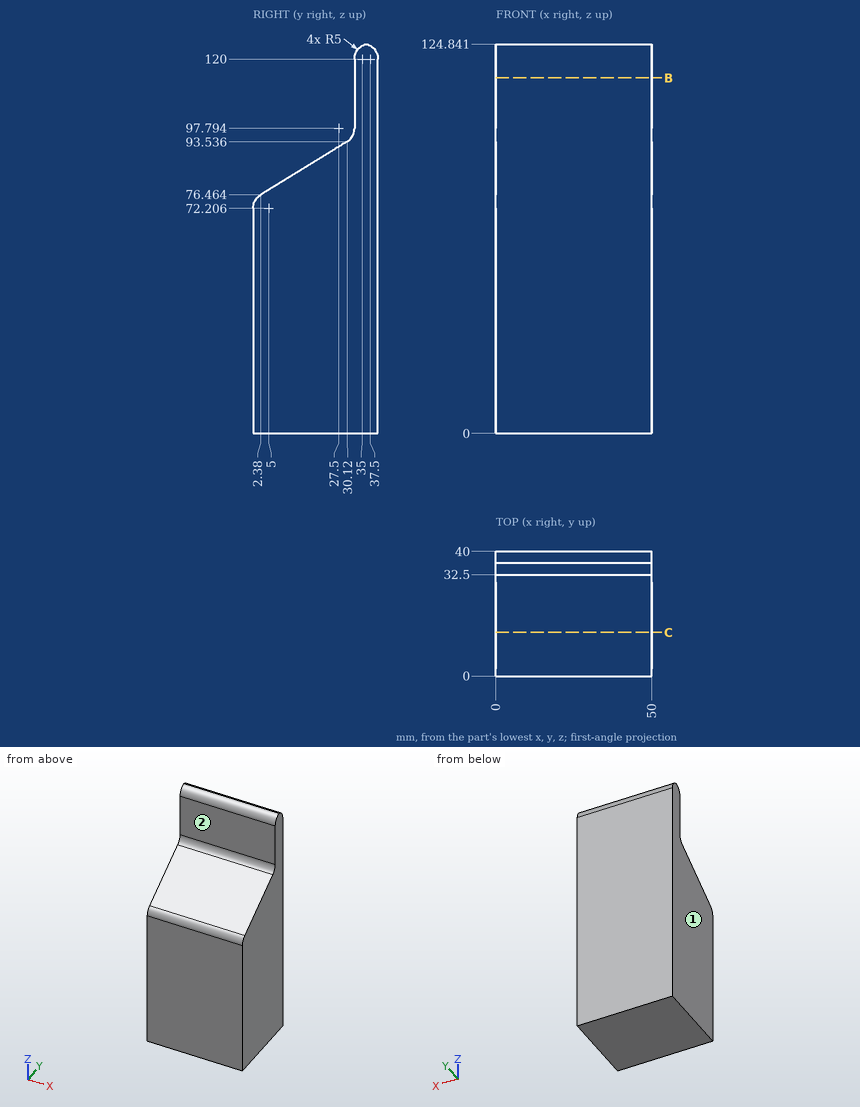
Job drawing, mm, ordinate dimensions from the low corner. One solid piece. A direction names the side the tool comes from. Round coordinates to 2 decimals unless told otherwise and drop trailing zeros. Loops run counter-clockwise (first coordinate to the right, second up) from the corner with the lowest first, then second, coordinate; pieces in that order, holes last. Notation, with made-up numbers: M -36,36.5 L -19,36.5 A13 cw -19,58.5 Z; hole C -22,73.5 d11. An arc over 180 degrees is marked long. Answer as CSV lines item,"result".
1. Cut at B-B on z = 114. Write the cut outline in (x, y).
Resolved:
outline,"M 0,32.5 L 50,32.5 L 50,40 L 0,40 Z"
2. Flat gauge pins, fed straight in: P1, Ø10, axis at x = 44.5, y = 32, coming from the +Z side; P2, Ø5, axis at y = 21.5, z = 35, coming from the -X side; P3, Ø11, axis at x = 19, z = 112.5, coming from the -Y side. Where does each tip first touch, or does it go through?
Resolved:
P1,"stops at z = 124.84"
P2,"stops at x = 0"
P3,"stops at y = 32.5"
3. Cut at C-C on y = 14. Write the cut outline in (x, z) (1 decimal).
Resolved:
outline,"M 0,0 L 50,0 L 50,83.6 L 0,83.6 Z"
4. Wall check: probe 1 along Y at (x, z) = (18, 118); probe 2 along Z at (x, y) = (34, 8.5); probe 3 along Z at (x, y) = (37, 12) (1 decimal). Give the ranges that are in metal, low to high. Write a range as [from, to].
Resolved:
probe 1,"y = [32.5, 40]"
probe 2,"z = [0, 80.23]"
probe 3,"z = [0, 82.4]"
5. 3-axis set-ups, long thin cutter, end or side, ignore diameter. For the marked faces 1 and 2: which of +Z, -Z, +X, -X, +Y, -Y reach the whole face in a straight line?
Resolved:
face 1,"+Z, -Z, -X, +Y, -Y"
face 2,"+Z, +X, -X, -Y"
